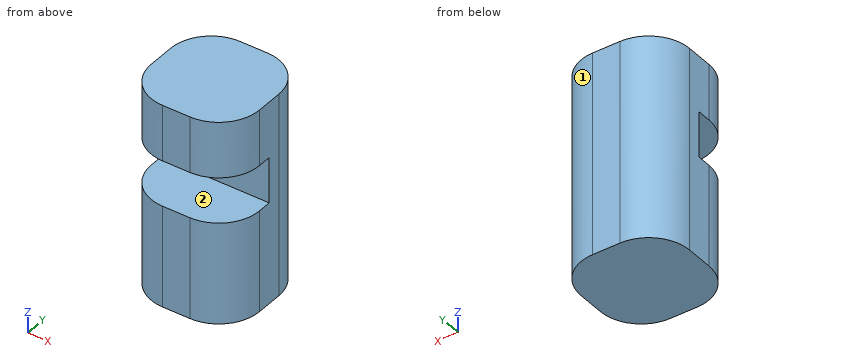
```python
from build123d import *

# Parameters (mm, degrees)
F0_W     = 800
F0_H     = 800
F1_DEPTH = 1500
F2_W     = 800
F2_H     = 336.829662323
F3_DEPTH = 400
F4_R     = 300


with BuildPart() as f1:
    # F0 (on Top) → F1 (new body)
    with BuildSketch(Plane.XY):
        with Locations((-4.4129546732, -53.8649755846)):
            Rectangle(F0_W, F0_H)
    extrude(amount=F1_DEPTH)

    # F2 (on face) → F3 (cut)
    with BuildSketch(Plane.XZ.offset(453.8649755846)):
        with Locations((-4.4129546732, 918.4148311615)):
            Rectangle(F2_W, F2_H)
    extrude(amount=-F3_DEPTH, mode=Mode.SUBTRACT)

    # F4
    f4_edges = [f1.edges().sort_by_distance(p)[0] for p in [
        (-404.412955, 346.135024, 750),
        (395.587045, 346.135024, 750),
        (-404.412955, -453.864976, 1293.414831),
        (-404.412955, -453.864976, 375),
        (395.587045, -453.864976, 1293.414831),
        (395.587045, -453.864976, 375),
    ]]
    fillet(f4_edges, radius=F4_R)


solid = f1.part
```
Input: part model. Units: mm. Frame: model coordinates. Face numbers are marked on the shaded views. A direction names the side the tool comes from. Coordinates: 2 decimals unless noted, no trailing zeros. Order: outer loops, then holes, each group sorted by start corner. A loop starts at its lowest first (then second) coordinate and runs counter-clockwise, first axis right, second up. Notation, with made-up numbers: (88, 64) - (113, 64) arc R17 cw to (113, 86) - close; hole circle Ø9 at (74.5, -9). An arc over 180 degrees is marked (long way). Put each result on its own line as item: value.
1. Reachability of the marked faces 1 and 2 from +Z, -Z, +X, -X, +Y, -Y: full face, straight path, thin tool, end or side. Return the list, or none.
Report:
face 1: +Z, -Z, +X, +Y
face 2: +X, -X, -Y
2. Cut plane C-C on z = 687. Return the cut outline in (x, y), then the cut area to 3 significant figures.
Report:
outline: (-404.41, -153.86) arc R300 ccw to (-104.41, -453.86) - (95.59, -453.86) arc R300 ccw to (395.59, -153.86) - (395.59, 46.14) arc R300 ccw to (95.59, 346.14) - (-104.41, 346.14) arc R300 ccw to (-404.41, 46.14) - close
area: 563,000 mm2
3. Cut plane D-D on y = -263. Return the cut outline in (x, z).
Report:
outline: (-383.86, 0) - (375.03, 0) - (375.03, 750) - (-383.86, 750) - close; (-383.86, 1086.83) - (375.03, 1086.83) - (375.03, 1500) - (-383.86, 1500) - close
4. Contact query for flat-ended pins moving along their axis: pin 1 Ø10 at (x, z) = (138, 1342.5) entering from +Y; pin 2 Ø6 at (y, z) = (-208.5, 1081.5) entering from +X; pin 3 Ø5 at (y, z) = (161, 1137.5) entering from -X (3 decimals); pin 4 Ø6 at (x, z) = (186, 1060.5) entering from -Y (3 decimals). Output: stop coordinate, or through.
Report:
pin 1: stops at y = 343.79
pin 2: passes through
pin 3: stops at x = -382.575
pin 4: stops at y = -53.865
5. Line query: line 1 along Z through (x, y) = (292.5, -78); line 2 along Y through (x, z) = (-97, 864.5); line 3 along Y through (x, z) = (-340.5, 1253). Output: solid intervals per line, ascending.
Report:
line 1: z = 0 to 750, 1086.83 to 1500
line 2: y = -53.86 to 346.14
line 3: y = -338.97 to 231.24
6. Cut plane A-A on y = -80.5. Return the cut outline in (x, z).
Report:
outline: (-404.41, 0) - (395.59, 0) - (395.59, 750) - (-404.41, 750) - close; (-404.41, 1086.83) - (395.59, 1086.83) - (395.59, 1500) - (-404.41, 1500) - close
7. Cut plane B-B on x = 16.5. Return the cut outline in (y, z), then the cut area to 3 significant figures.
Report:
outline: (-453.86, 0) - (346.14, 0) - (346.14, 1500) - (-453.86, 1500) - (-453.86, 1086.83) - (-53.86, 1086.83) - (-53.86, 750) - (-453.86, 750) - close
area: 1,070,000 mm2
